Design review of the part shown in the three views and the two pictorial views. Dimensions are in mm from the part's minimum x, y and z. A direction names the side the tool comes from. Give positions to 0.01 mm unless a question says otherwise; leave off trailing zeros. Order: outer loops, then holes, each group sorted by start corner. A loop starts at its lowest first (then second) coordinate and runs counter-clockwise, first axis right, second up. Notation, with made-up numbers: (-18, -33) - (15, -33) arc R25 ccw to (15, 6) - close; hole circle Ø2 at (-38.5, 58.5). An arc over 180 degrees is marked (long way). Write each question's results on one line, items separated by ' | '. Start each with the question number.
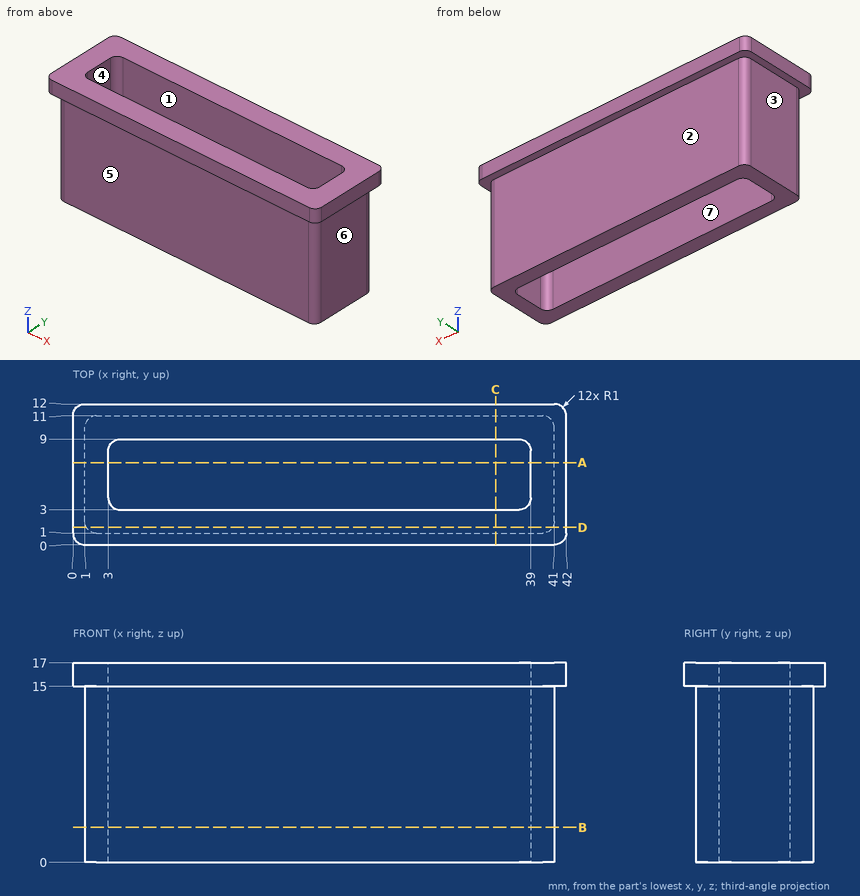
Q1. For line 1 (Y direction, x = 22, z = 8.75); line 2 (X direction, y = 7, z = 5.25); line 3 (X direction, y = 1.25, z = 1), list the stretches that pass through material, from the lowest coordinate up. Write a range as [from, to].
Q2. Add section D-D (y = 1.5). Give the boundary of the cut face in (x, z), plus the area to 3 significant figures.
Q3. Draft analysis for pull direction X (two halves, no side actions). For the marked faces 4, 5, 6 and 7, state which applies: pulls with the +X half, pulls with the -X half, needs draft (parallel to the pull), parting line crosses it, or undercut.
Q4. Add section A-A (y = 7). Give the boundary of the cut face in (x, z), plus the area to 3 significant figures.
Q5. Add section C-C (x = 36). Give the boundary of the cut face in (y, z), plus the area to 3 significant figures.
Q6. Insertion check: pin 1 Ø2 at (y, z) = (5, 9) entering from -X; pin 2 Ø4 at (y, z) = (7, 5) entering from +X; pin 3 Ø1 at (x, z) = (15, 6.5) entering from +Y. Each pin has a flat end and moves straight along its axis. Give the tip position at first contact, or say it passes through.
Q7. Add section B-B (z = 3). Give the boundary of the cut face in (x, y), plus the area to 3 significant figures.
Q8. Machinability: for the marked faces 1, 2 and 3, which of the approach directions +Z, -Z, +X, -X, +Y, -Y give a long, thin tool a straight path to every point of the face, cutting with its end or side? Answer none if there is none.
Verdict:
1) line 1: y = [1, 3], [9, 11] | line 2: x = [1, 3], [39, 41] | line 3: x = [1.34, 40.66]
2) outline: (0, 15) - (1.13, 15) - (1.13, 0) - (40.87, 0) - (40.87, 15) - (42, 15) - (42, 17) - (0, 17) - close | area: 680 mm2
3) face 4: undercut | face 5: needs draft | face 6: pulls with the +X half | face 7: undercut
4) outline: (0, 15) - (1, 15) - (1, 0) - (3, 0) - (3, 17) - (0, 17) - close; (39, 0) - (41, 0) - (41, 15) - (42, 15) - (42, 17) - (39, 17) - close | area: 72.0 mm2
5) outline: (0, 15) - (1, 15) - (1, 0) - (3, 0) - (3, 17) - (0, 17) - close; (9, 0) - (11, 0) - (11, 15) - (12, 15) - (12, 17) - (9, 17) - close | area: 72.0 mm2
6) pin 1: stops at x = 1 | pin 2: stops at x = 41 | pin 3: stops at y = 11
7) outline: (1, 2) arc R1 ccw to (2, 1) - (40, 1) arc R1 ccw to (41, 2) - (41, 10) arc R1 ccw to (40, 11) - (2, 11) arc R1 ccw to (1, 10) - close; hole (3, 4) arc R1 ccw to (4, 3) - (38, 3) arc R1 ccw to (39, 4) - (39, 8) arc R1 ccw to (38, 9) - (4, 9) arc R1 ccw to (3, 8) - close | area: 184 mm2
8) face 1: +Z, -Z | face 2: -Z, +X, -X, +Y | face 3: -Z, -X, +Y, -Y
